Read the model definition and answer for the solid it produces. Units are mm, in the model's axes. A direction names the side the tool comes from. Coordinates: 2 decimals unless noted, no trailing zeros. Write each loop counter-clockwise with the first axis right and the second up, starting at its lowest first coordinate (ties: lowest second). Pieces come first, ordered by that corner, then holes. Notation, with made-up numbers: (28.25, -33) - (54.25, -33) arc R26 ccw to (54.25, -13) - close; hole circle Ø11 at (16, 79.5). An arc over 180 degrees is marked (long way). Return JSON: item names as keys, results as strings.
```python
from build123d import *

# Parameters (mm, degrees)
F1_DEPTH = 2.75


# Not quite as in the source:
# - a fillet or chamfer that OpenCascade refuses, or shapes differently, is made with other operations: its cross-section is extruded or revolved along the edge and cut away or added


with BuildPart() as f1:
    # F0 (on Top) → F1 (new body)
    with BuildSketch(Plane.XY):
        with BuildLine():
            ThreePointArc((-15.79, 16.88), (-14.7293398282, 16.4406601718), (-14.29, 15.38))
            Line((-14.29, 15.38), (-14.29, 13.88))
            Line((-14.29, 13.88), (-12.3530682288, 13.88))
            ThreePointArc((-12.3530682288, 13.88), (-12.1191013265, 14.6138388362), (-12.04, 15.38))
            ThreePointArc((-12.04, 15.38), (-12.1191013265, 16.1461611638), (-12.3530682288, 16.88))
            Line((-12.3530682288, 16.88), (-15.79, 16.88))
        make_face()
        with BuildLine():
            ThreePointArc((-17.29, 15.38), (-16.8506601718, 16.4406601718), (-15.79, 16.88))
            Line((-15.79, 16.88), (-12.3530682288, 16.88))
            ThreePointArc((-12.3530682288, 16.88), (-18.4416504294, 18.0316504294), (-17.29, 11.9430682288))
            Line((-17.29, 11.9430682288), (-17.29, 15.38))
        make_face()
        with BuildLine():
            Line((-14.29, 13.88), (-15.79, 13.88))
            ThreePointArc((-15.79, 13.88), (-16.8506601718, 14.3193398282), (-17.29, 15.38))
            Line((-17.29, 15.38), (-17.29, 11.9430682288))
            ThreePointArc((-17.29, 11.9430682288), (-15.79, 11.63), (-14.29, 11.9430682288))
            Line((-14.29, 11.9430682288), (-14.29, 13.88))
        make_face()
        with BuildLine():
            Line((12.3530682288, 16.88), (-12.3530682288, 16.88))
            ThreePointArc((-12.3530682288, 16.88), (-12.1191013265, 16.1461611638), (-12.04, 15.38))
            ThreePointArc((-12.04, 15.38), (-12.1191013265, 14.6138388362), (-12.3530682288, 13.88))
            Line((-12.3530682288, 13.88), (12.3530682288, 13.88))
            ThreePointArc((12.3530682288, 13.88), (12.04, 15.38), (12.3530682288, 16.88))
        make_face()
        with BuildLine():
            Line((-14.29, -11.9430682288), (-14.29, 11.9430682288))
            ThreePointArc((-14.29, 11.9430682288), (-15.79, 11.63), (-17.29, 11.9430682288))
            Line((-17.29, 11.9430682288), (-17.29, -11.9430682288))
            ThreePointArc((-17.29, -11.9430682288), (-15.79, -11.63), (-14.29, -11.9430682288))
        make_face()
        with BuildLine():
            Line((15.79, 16.88), (12.3530682288, 16.88))
            ThreePointArc((12.3530682288, 16.88), (12.04, 15.38), (12.3530682288, 13.88))
            Line((12.3530682288, 13.88), (14.29, 13.88))
            Line((14.29, 13.88), (14.29, 15.38))
            ThreePointArc((14.29, 15.38), (14.7293398282, 16.4406601718), (15.79, 16.88))
        make_face()
        with BuildLine():
            ThreePointArc((19.54, 15.38), (16.5561611638, 19.0508986735), (12.3530682288, 16.88))
            Line((12.3530682288, 16.88), (15.79, 16.88))
            ThreePointArc((15.79, 16.88), (16.8506601718, 16.4406601718), (17.29, 15.38))
            Line((17.29, 15.38), (17.29, 11.9430682288))
            ThreePointArc((17.29, 11.9430682288), (18.9274750995, 13.3260404094), (19.54, 15.38))
        make_face()
        with BuildLine():
            Line((-14.29, -13.88), (-14.29, -11.9430682288))
            ThreePointArc((-14.29, -11.9430682288), (-15.79, -11.63), (-17.29, -11.9430682288))
            Line((-17.29, -11.9430682288), (-17.29, -15.38))
            ThreePointArc((-17.29, -15.38), (-16.8506601718, -14.3193398282), (-15.79, -13.88))
            Line((-15.79, -13.88), (-14.29, -13.88))
        make_face()
        with BuildLine():
            Line((-17.29, -15.38), (-17.29, -11.9430682288))
            ThreePointArc((-17.29, -11.9430682288), (-18.4416504294, -18.0316504294), (-12.3530682288, -16.88))
            Line((-12.3530682288, -16.88), (-15.79, -16.88))
            ThreePointArc((-15.79, -16.88), (-16.8506601718, -16.4406601718), (-17.29, -15.38))
        make_face()
        with BuildLine():
            Line((12.3530682288, -13.88), (-12.3530682288, -13.88))
            ThreePointArc((-12.3530682288, -13.88), (-12.1191013265, -14.6138388362), (-12.04, -15.38))
            ThreePointArc((-12.04, -15.38), (-12.1191013265, -16.1461611638), (-12.3530682288, -16.88))
            Line((-12.3530682288, -16.88), (12.3530682288, -16.88))
            ThreePointArc((12.3530682288, -16.88), (12.04, -15.38), (12.3530682288, -13.88))
        make_face()
        with BuildLine():
            ThreePointArc((-12.04, -15.38), (-12.1191013265, -14.6138388362), (-12.3530682288, -13.88))
            Line((-12.3530682288, -13.88), (-14.29, -13.88))
            Line((-14.29, -13.88), (-14.29, -15.38))
            ThreePointArc((-14.29, -15.38), (-14.7293398282, -16.4406601718), (-15.79, -16.88))
            Line((-15.79, -16.88), (-12.3530682288, -16.88))
            ThreePointArc((-12.3530682288, -16.88), (-12.1191013265, -16.1461611638), (-12.04, -15.38))
        make_face()
        with BuildLine():
            Line((14.29, 13.88), (14.29, 11.9430682288))
            ThreePointArc((14.29, 11.9430682288), (15.79, 11.63), (17.29, 11.9430682288))
            Line((17.29, 11.9430682288), (17.29, 15.38))
            ThreePointArc((17.29, 15.38), (16.8506601718, 14.3193398282), (15.79, 13.88))
            Line((15.79, 13.88), (14.29, 13.88))
        make_face()
        with BuildLine():
            ThreePointArc((17.29, 11.9430682288), (15.79, 11.63), (14.29, 11.9430682288))
            Line((14.29, 11.9430682288), (14.29, -11.9430682288))
            ThreePointArc((14.29, -11.9430682288), (15.79, -11.63), (17.29, -11.9430682288))
            Line((17.29, -11.9430682288), (17.29, 11.9430682288))
        make_face()
        with BuildLine():
            Line((14.29, -13.88), (12.3530682288, -13.88))
            ThreePointArc((12.3530682288, -13.88), (12.04, -15.38), (12.3530682288, -16.88))
            Line((12.3530682288, -16.88), (15.79, -16.88))
            ThreePointArc((15.79, -16.88), (14.7293398282, -16.4406601718), (14.29, -15.38))
            Line((14.29, -15.38), (14.29, -13.88))
        make_face()
        with BuildLine():
            ThreePointArc((17.29, -11.9430682288), (15.79, -11.63), (14.29, -11.9430682288))
            Line((14.29, -11.9430682288), (14.29, -13.88))
            Line((14.29, -13.88), (15.79, -13.88))
            ThreePointArc((15.79, -13.88), (16.8506601718, -14.3193398282), (17.29, -15.38))
            Line((17.29, -15.38), (17.29, -11.9430682288))
        make_face()
        with BuildLine():
            Line((15.79, -16.88), (12.3530682288, -16.88))
            ThreePointArc((12.3530682288, -16.88), (16.5561611638, -19.0508986735), (19.54, -15.38))
            ThreePointArc((19.54, -15.38), (18.9274750995, -13.3260404094), (17.29, -11.9430682288))
            Line((17.29, -11.9430682288), (17.29, -15.38))
            ThreePointArc((17.29, -15.38), (16.8506601718, -16.4406601718), (15.79, -16.88))
        make_face()
        with BuildLine():
            Line((-14.29, 13.88), (-14.29, 15.38))
            ThreePointArc((-14.29, 15.38), (-14.7293398282, 14.3193398282), (-15.79, 13.88))
            Line((-15.79, 13.88), (-14.29, 13.88))
        make_face()
        with BuildLine():
            Line((-12.3530682288, 13.88), (-14.29, 13.88))
            Line((-14.29, 13.88), (-14.29, 11.9430682288))
            ThreePointArc((-14.29, 11.9430682288), (-13.1383495706, 12.7283495706), (-12.3530682288, 13.88))
        make_face()
        with BuildLine():
            Line((14.29, 13.88), (12.3530682288, 13.88))
            ThreePointArc((12.3530682288, 13.88), (13.1383495706, 12.7283495706), (14.29, 11.9430682288))
            Line((14.29, 11.9430682288), (14.29, 13.88))
        make_face()
        with BuildLine():
            Line((14.29, 15.38), (14.29, 13.88))
            Line((14.29, 13.88), (15.79, 13.88))
            ThreePointArc((15.79, 13.88), (14.7293398282, 14.3193398282), (14.29, 15.38))
        make_face()
        with BuildLine():
            Line((-14.29, -15.38), (-14.29, -13.88))
            Line((-14.29, -13.88), (-15.79, -13.88))
            ThreePointArc((-15.79, -13.88), (-14.7293398282, -14.3193398282), (-14.29, -15.38))
        make_face()
        with BuildLine():
            ThreePointArc((-12.3530682288, -13.88), (-13.1383495706, -12.7283495706), (-14.29, -11.9430682288))
            Line((-14.29, -11.9430682288), (-14.29, -13.88))
            Line((-14.29, -13.88), (-12.3530682288, -13.88))
        make_face()
        with BuildLine():
            Line((15.79, -13.88), (14.29, -13.88))
            Line((14.29, -13.88), (14.29, -15.38))
            ThreePointArc((14.29, -15.38), (14.7293398282, -14.3193398282), (15.79, -13.88))
        make_face()
        with BuildLine():
            ThreePointArc((14.29, -11.9430682288), (13.1383495706, -12.7283495706), (12.3530682288, -13.88))
            Line((12.3530682288, -13.88), (14.29, -13.88))
            Line((14.29, -13.88), (14.29, -11.9430682288))
        make_face()
    extrude(amount=F1_DEPTH)

    # F2: chamfer of 2 on 4 edges, made by hand

    # F2_s1 → F2_t2 (revolve, cut)
    with BuildSketch(Plane.XZ.offset(-15.38)):
        Polygon((-14.29, 0.75), (-12.29, 2.75), (-14.29, 2.75), align=None)
    revolve(axis=Axis((-15.79, 15.38, 2.75), (0, 0, -1)), mode=Mode.SUBTRACT)

    # F2_s3 → F2_t4 (revolve, cut)
    with BuildSketch(Plane.YZ.offset(15.79)):
        Polygon((13.88, 0.75), (11.88, 2.75), (13.88, 2.75), align=None)
    revolve(axis=Axis((15.79, 15.38, 2.75), (0, 0, -1)), mode=Mode.SUBTRACT)

    # F2_s5 → F2_t6 (revolve, cut)
    with BuildSketch(Plane.XZ.offset(15.38)):
        Polygon((14.29, 0.75), (12.29, 2.75), (14.29, 2.75), align=None)
    revolve(axis=Axis((15.79, -15.38, 2.75), (0, 0, -1)), mode=Mode.SUBTRACT)

    # F2_s7 → F2_t8 (revolve, cut)
    with BuildSketch(Plane.YZ.offset(-15.79)):
        Polygon((-13.88, 0.75), (-11.88, 2.75), (-13.88, 2.75), align=None)
    revolve(axis=Axis((-15.79, -15.38, 2.75), (0, 0, -1)), mode=Mode.SUBTRACT)


solid = f1.part
```
(1) Which of the six approach directions +Z, -Z, +X, -X, +Y, -Y give full straight-line access (tool end or side, diameter ignored) to faces 4 (the face through (0, 16.88, 1)), 5 (the face through (0, -16.88, 1)), 6 (the face through (13.152, -12.715, 1.356))?
Answer:
{"face 4": "+Z, -Z, +Y", "face 5": "+Z, -Z, -Y", "face 6": "+Z, -Z"}
(2) Determine the mould class of faces 1 (the face through (-0.1, 14.3, 2.75)), 2 (the face through (17.29, 0, 1)), 3 (the face through (14.29, 0, 1)) for opening direction X: +X half, -X half, draft (parallel to the pull), parting line (faces both ways), or undercut.
Answer:
{"face 1": "draft", "face 2": "+X half", "face 3": "undercut"}
(3) A cutting plane is placed at B-B (z = 1.6). Determine the outline of the cut face in (x, y), and give its area (3 significant figures).
Answer:
{"outline": "(-17.29, -11.94) arc R3.75 ccw (long way) to (-12.35, -16.88) - (12.35, -16.88) arc R3.75 ccw (long way) to (17.29, -11.94) - (17.29, 11.94) arc R3.75 ccw (long way) to (12.35, 16.88) - (-12.35, 16.88) arc R3.75 ccw (long way) to (-17.29, 11.94) - close; hole circle Ø4.7 at (-15.79, -15.38); hole circle Ø4.7 at (-15.79, 15.38); hole (-14.29, -11.94) arc R3.75 cw to (-12.35, -13.88) - (12.35, -13.88) arc R3.75 cw to (14.29, -11.94) - (14.29, 11.94) arc R3.75 cw to (12.35, 13.88) - (-12.35, 13.88) arc R3.75 cw to (-14.29, 11.94) - close; hole circle Ø4.7 at (15.79, -15.38); hole circle Ø4.7 at (15.79, 15.38)", "area": "394 mm²"}
(4) A cutting plane is placed at A-A (y = -2.5). Determine the outline of the cut face in (x, z).
Answer:
{"outline": "(-17.29, 0) - (-14.29, 0) - (-14.29, 2.75) - (-17.29, 2.75) - close; (14.29, 0) - (17.29, 0) - (17.29, 2.75) - (14.29, 2.75) - close"}
(5) A cutting plane is placed at C-C (x = 3). Determine the outline of the cut face in (y, z), and give its area (3 significant figures).
Answer:
{"outline": "(-16.88, 0) - (-13.88, 0) - (-13.88, 2.75) - (-16.88, 2.75) - close; (13.88, 0) - (16.88, 0) - (16.88, 2.75) - (13.88, 2.75) - close", "area": "16.5 mm²"}
(6) Straight lines are drawn through the part: line 1 (X direction, y = -15.5, z = 0.2); line 2 (Y direction, x = 4.5, z = 1.8); line 3 (X direction, y = 3.5, z = 2.25). For each, find the intervals that lie inside material, in ascending order. Write a range as from..to.
Answer:
{"line 1": "-19.54..-17.29, -14.29..14.29, 17.29..19.54", "line 2": "-16.88..-13.88, 13.88..16.88", "line 3": "-17.29..-14.29, 14.29..17.29"}
(7) Flat-ended cylindrical pins translate along their axes: P1, Ø1.4, axis at y = -1.5, z = 1, coming from the -X side; P2, Ø0.8, axis at x = 4, z = 1, coming from the +Y side; P3, Ø1.4, axis at x = 2.5, z = 2, coming from the -Y side. Find the tip coordinate at first contact, or state that the pin passes through.
Answer:
{"P1": "x = -17.29", "P2": "y = 16.88", "P3": "y = -16.88"}
(8) A cutting plane is placed at D-D (x = 15). State how many separate pieces and enclosed holes the cut face has, and give its area (3 significant figures).
Answer:
{"separate pieces": "3", "enclosed holes": "0", "area": "82.0 mm²"}
